Autodesk Inventor part; units mm, degrees
ref_plane "YZ Plane" through (0, 0, 0) normal (1, 0, 0) x (0, 1, 0)
ref_plane "XZ Plane" through (0, 0, 0) normal (0, 1, 0) x (-1, 0, 0)
ref_plane "XY Plane" through (0, 0, 0) normal (0, 0, 1) x (1, 0, 0)
sketch "Sketch1" plane through (0, 0, 0) normal (0, 0, 1) x (1, 0, 0)
  circle A0 centre (0, 0) radius 76.2
  dimension "tubeDiameter" = 152.4
extrude "Extrusion1" add sketch "Sketch1" along normal mid plane 438.15
sketch "Sketch2" plane through (0, 0, -219.075) normal (0, 0, -1) x (-1, 0, 0)
  circle A0 centre (0, 0) radius 73.025
  dimension "d6" = 146.05
extrude "Extrusion2" cut sketch "Sketch2" against normal blind 406.4
sketch "Sketch3" plane through (0, 0, 219.075) normal (0, 0, 1) x (1, 0, 0)
  circle A0 centre (0, 0) radius 82.55
  circle A1 centre (0, 0) radius 76.2
  dimension "d9" = 165.1
extrude "Extrusion3" add sketch "Sketch3" against normal blind 25.4
sketch "Sketch4" plane through (0, 0, -219.075) normal (0, 0, -1) x (-1, 0, 0)
  circle A0 centre (0, 0) radius 76.2
  circle A1 centre (0, 0) radius 82.55
extrude "Extrusion4" add sketch "Sketch4" against normal blind 25.4
sketch "Sketch7" plane through (0, 0, 219.075) normal (0, 0, 1) x (1, 0, 0)
  circle A0 centre (0, 0) radius 82.55
  circle A1 centre (0, 0) radius 82.55
extrude "Extrusion6" cut sketch "Sketch7" against normal blind 311.15
properties part number "trussTelescopeTubeFront" material "Aluminum 6061"
Part model, mm, in its own coordinate system. Round coordinates to 2 decimals unless told otherwise and drop trailing zeros. Order: outer loops, then holes, each group sorted by start corner. A loop starts at its lowest first (then second) coordinate and runs counter-clockwise, first axis right, second up. Notation, with made-up numbers: (1.5, -23) -> (38.5, -23) arc R25 cw to (38.5, 7) -> close; hole circle Ø6 at (-10, -19.5). An arc over 180 degrees is marked (long way). Put each result on its own line as item: value.
Q1. Band-saw the part on C-C (z = -166). Give the cut face in (x, y) (3 decimals), and give its area (3 significant figures).
From the geometry:
outline: circle Ø152.4 at (0, 0); hole circle Ø146.05 at (0, 0)
area: 1,490 mm2
Q2. Band-saw the part on A-A (y = 0). Give the cut face in (x, z) (3 decimals), and give its area (3 significant figures).
From the geometry:
outline: (-82.55, -219.075) -> (-73.025, -219.075) -> (-73.025, -92.075) -> (-76.2, -92.075) -> (-76.2, -193.675) -> (-82.55, -193.675) -> close; (73.025, -219.075) -> (82.55, -219.075) -> (82.55, -193.675) -> (76.2, -193.675) -> (76.2, -92.075) -> (73.025, -92.075) -> close
area: 1,130 mm2
Q3. Pull direction X, two halves, no side cores. Call faces 1 (the face through (-24, -73, -193.675)), 2 (the face through (-69.653, 21.935, -156.464)), 3 (the face through (-60.47, -46.367, -142.164)): pulls with the +X half, pulls with the -X half, needs draft (parallel to the pull), parting line crosses it, or undercut.
From the geometry:
face 1: needs draft
face 2: undercut
face 3: parting line crosses it
Q4. Pin check, flat tips, straight feed: pin 1 Ø12 at (x, z) = (31.5, -113) entering from -Y; pin 2 Ø3 at (x, z) = (54, -191) entering from -Y; pin 3 Ø12 at (x, z) = (51, -153) entering from -Y. Stop position of each tip, or through.
From the geometry:
pin 1: stops at y = -71.81
pin 2: stops at y = -55.23
pin 3: stops at y = -61.49
Q5. Wall check: line 1 (Y direction, x = 0, z = -193.5) (3 decimals); line 2 (Z direction, x = -61, y = 47.5) (3 decimals); line 3 (X direction, y = -31, z = -170). Give the ranges that are in metal, low to high. Write a range as [from, to].
From the geometry:
line 1: y = [-76.2, -73.025], [73.025, 76.2]
line 2: z = [-219.075, -193.675]
line 3: x = [-69.61, -66.12], [66.12, 69.61]
